Can you work these out from the drawing? Everything is in mm from the part's minimum corner. A direction names the side the tool comes from. Give positions to 0.01 mm unless a question says otherwise; leave off trailing zeros. Write each loop counter-clockwise with the first axis right and the second up, starting at its lowest first coordinate (ties: lowest second). Pieces come first, ordered by that corner, then holes. Notation, with made-up numbers: (16.5, 88) - (59.5, 88) arc R22 ccw to (59.5, 112) - close; hole circle Ø3 at (62.25, 61). An arc over 180 degrees is marked (long way). Write each question's results on one line, items separated by ' | '. Start each with the question number.
Item 1: We'd pull the mould along Z, two halves only. Please class the marked faces 4, 5 and 6: +Z half, -Z half, draft (parallel to the pull), parting line (faces both ways), or undercut.
Item 2: Which directions (+Z, -Z, +X, -X, +Y, -Y) give clear straight access to the entire face, cutting with the end or side of a thin tool? Please do the marked faces 1, 2 and 3.
Item 3: Please list where these lines run through material, in increasing order: line 1 along Y through (x, z) = (33.5, 25); line 2 along Y through (x, z) = (21, 25); line 3 along X through (y, z) = (33, 37).
Item 4: Suppose I cut it at B-B on x = 25. List the corners of the cut face in (y, z) for me.
Item 5: Suppose I cut it at A-A on z = 25. List the corners of the cut face in (x, y) for me.
Item 6: Suppose I cut it at C-C on y = 70. List the corners of the cut face in (x, z) for me.
Item 7: Will these pins go through, and if not, where does the flat tip stop? P1, Ø12, axis at x = 28, z = 21, coming from the -Y side; P2, Ø6, axis at x = 3.5, z = 27.5, coming from the +Y side; P3, Ø12, axis at y = 40, z = 23.5, coming from the -X side; P4, Ø6, axis at x = 25, z = 25, coming from the -Y side.
Item 8: Suppose I cut it at D-D on z = 17. List the corners of the cut face in (x, y) for me.
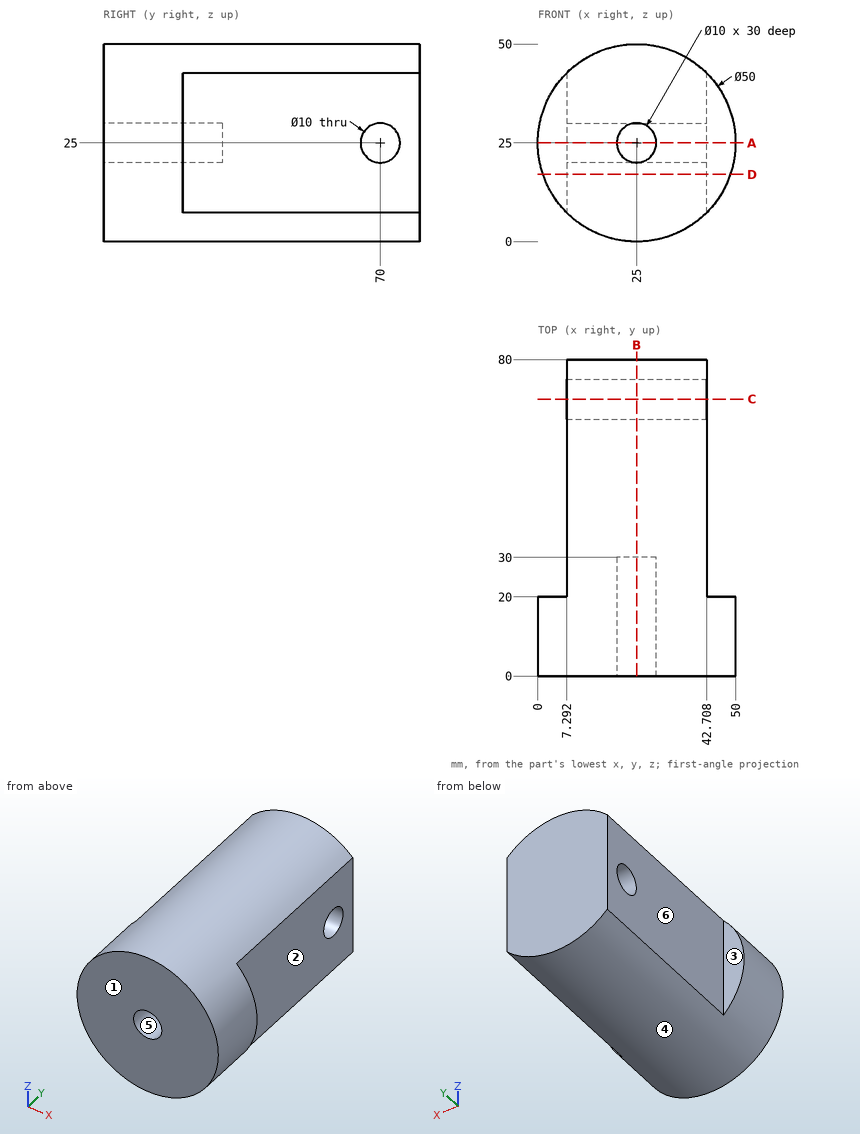
Checked values:
1) face 4: parting line | face 5: undercut | face 6: draft
2) face 1: +Z, -Z, +X, -X, -Y | face 2: +Z, -Z, +X, +Y | face 3: +Z, -Z, -X, +Y
3) line 1: y = 0 to 65, 75 to 80 | line 2: y = 30 to 65, 75 to 80 | line 3: x = 7.29 to 42.71
4) outline: (0, 0) - (80, 0) - (80, 50) - (0, 50) - (0, 30) - (30, 30) - (30, 20) - (0, 20) - close; hole circle Ø10 at (70, 25)
5) outline: (0, 0) - (20, 0) - (20, 30) - (30, 30) - (30, 0) - (50, 0) - (50, 20) - (42.71, 20) - (42.71, 65) - (7.29, 65) - (7.29, 20) - (0, 20) - close; (7.29, 75) - (42.71, 75) - (42.71, 80) - (7.29, 80) - close
6) outline: (7.29, 7.35) arc R25 ccw to (42.71, 7.35) - (42.71, 20) - (7.29, 20) - close; (7.29, 30) - (42.71, 30) - (42.71, 42.65) arc R25 ccw to (7.29, 42.65) - close
7) P1: stops at y = 0 | P2: stops at y = 20 | P3: stops at x = 7.29 | P4: stops at y = 30
8) outline: (1.31, 0) - (48.69, 0) - (48.69, 20) - (42.71, 20) - (42.71, 80) - (7.29, 80) - (7.29, 20) - (1.31, 20) - close
